from build123d import *

# Parameters (mm, degrees)
SKETCH1_R           = 15
BOSS_EXTRUDE1_DEPTH = 10
SKETCH2_R           = 4.9
BOSS_EXTRUDE2_DEPTH = 15
CUT_EXTRUDE1_DEPTH  = 4


with BuildPart() as part:
    # Sketch1 → Boss-Extrude1 (new body)
    with BuildSketch(Plane(origin=(0, 0, 0), x_dir=(1, 0, 0), z_dir=(0, 1, 0))):
        Circle(SKETCH1_R)
    extrude(amount=BOSS_EXTRUDE1_DEPTH)

    # Sketch2 → Boss-Extrude2 (add)
    with BuildSketch(Plane(origin=(0, 10, 0), x_dir=(1, 0, 0), z_dir=(0, 1, 0))):
        Circle(SKETCH2_R)
    extrude(amount=BOSS_EXTRUDE2_DEPTH)

    # Sketch3 → Cut-Extrude1 (cut)
    with BuildSketch(Plane(origin=(0, 25, 0), x_dir=(1, 0, 0), z_dir=(0, 1, 0))):
        with BuildLine():
            Line((-4.9, 0), (0, 4.9))
            ThreePointArc((0, 4.9), (-3.464823228, 3.464823228), (-4.9, 0))
        make_face()
    extrude(amount=-CUT_EXTRUDE1_DEPTH, mode=Mode.SUBTRACT)


solid = part.part
The model under review builds one solid part; all positions refer to its coordinate system, in mm. A direction names the side the tool comes from. Give positions to 0.01 mm unless a question says otherwise; leave off trailing zeros. Order: outer loops, then holes, each group sorted by start corner. A loop starts at its lowest first (then second) coordinate and runs counter-clockwise, first axis right, second up. Notation, with made-up numbers: M 46,40 L 69,40 A22 cw 69,60 Z; hole C -11,36.25 d9. An arc over 180 degrees is marked long. Use one line per item in the form item = value. Start each with the question number.
Item 1: Insertion check: pin 1 Ø8 at (x, y) = (-11, 17.5) entering from -Z (1 decimal); pin 2 Ø2 at (y, z) = (18.5, -1.5) entering from -X; pin 3 Ø4 at (y, z) = (3.5, 6.5) entering from +X; pin 4 Ø1 at (x, y) = (6.5, 8.5) entering from +Z. Each pin has a flat end and moves straight along its axis. Give the tip position at first contact, or say it passes through.
Item 2: We need section B-B on z = 3. Give the boundary of the cut face in (x, y), plus the area to 3 significant figures.
Item 3: We need section C-C on x = -7. Give the boundary of the cut face in (y, z).
Item 4: We need section D-D on y = 3.25. Give the boundary of the cut face in (x, z), plus the area to 3 significant figures.
Item 5: For faces 1 (the flat face through (-2.5, 23, -2.4)), 2 (the flat face through (0, 25, 0)), 3 (the flat face through (-4, 10, -4)), list the 3-axis set-ups (+Z, -Z, +X, -X, +Y, -Y) from which the entire face can be reached by the end or side of a thin tool; tool diameter is ignored.
Item 6: We need section A-A on y = 23.5. Give the boundary of the cut face in (x, z).
Item 7: To check wall thickness, follow line 1 along Y through (x, z) = (-6.75, -13); line 2 along Z through (x, y) = (5.5, 3.5); line 3 along X through (y, z) = (7.5, -11.5). State the ranges of each line that lie inside material, in increasing order. Write a range as from..to.
Completed:
q1.pin_1 = through
q1.pin_2 = -4.87
q1.pin_3 = 14.31
q1.pin_4 = 13.75
q2.outline = M -14.7,0 L 14.7,0 L 14.7,10 L 3.87,10 L 3.87,25 L -3.87,25 L -3.87,10 L -14.7,10 Z
q2.area = 410 mm²
q3.outline = M 0,-13.27 L 10,-13.27 L 10,13.27 L 0,13.27 Z
q4.outline = C 0,0 d30
q4.area = 707 mm²
q5.face_1 = -Z, -X, +Y
q5.face_2 = +Z, -Z, +X, -X, +Y
q5.face_3 = +Y
q6.outline = M -4.9,0 L 0,-4.9 A4.9 ccw long Z
q7.line_1 = 0..10
q7.line_2 = -13.96..13.96
q7.line_3 = -9.63..9.63
